from build123d import *

# Parameters (mm, degrees)
SKETCH_1_W          = 38
SKETCH_1_H          = 20
EXTRUDE_1_DEPTH     = 10
SKETCH_2_R          = 2.025
CUT_EXTRUDE_1_DEPTH = 30.342801502
FILLET_1_R          = 0.5
SKETCH_3_R          = 2.5
CUT_EXTRUDE_2_DEPTH = 30.342801604
FILLET_2_R          = 1.5


with BuildPart() as part:
    # 草图1 → 凸台-拉伸1 (new, symmetric)
    with BuildSketch(Plane.XY):
        Rectangle(SKETCH_1_W, SKETCH_1_H)
        with BuildLine():
            Line((2.601020514, 1), (-2.601020514, 1))
            ThreePointArc((-2.601020514, 1), (-12.5, 0), (-2.601020514, -1))
            Line((-2.601020514, -1), (2.601020514, -1))
            ThreePointArc((2.601020514, -1), (12.5, 0), (2.601020514, 1))
        make_face(mode=Mode.SUBTRACT)
    extrude(amount=EXTRUDE_1_DEPTH, both=True)

    # 草图2 → 切除-拉伸1 (cut, through all)
    with BuildSketch(Plane(origin=(0, 10, 0), x_dir=(1, 0, 0), z_dir=(0, 1, 0))):
        with Locations(Location((-7.5, 0, 0), (0, 0, 180))):
            Circle(SKETCH_2_R)
        with Locations(Location((7.5, 0, 0), (0, 0, 180))):
            Circle(SKETCH_2_R)
    extrude(amount=-CUT_EXTRUDE_1_DEPTH, mode=Mode.SUBTRACT)

    # 圆角1
    fillet_1_edges = [part.edges().sort_by_distance(p)[0] for p in [
        (2.601020514, -1, 0),
        (2.601020514, 1, 0),
        (-2.601020514, 1, 0),
        (-2.601020514, -1, 0),
    ]]
    fillet(fillet_1_edges, radius=FILLET_1_R)

    # 草图3 → 切除-拉伸2 (cut, through all)
    with BuildSketch(Plane.XY.offset(10)):
        with Locations((0, 10)):
            Circle(SKETCH_3_R)
        with Locations((0, -10)):
            Circle(SKETCH_3_R)
    extrude(amount=-CUT_EXTRUDE_2_DEPTH, mode=Mode.SUBTRACT)

    # 圆角2
    fillet_2_edges = [part.edges().sort_by_distance(p)[0] for p in [
        (19, 0, 10),
        (-19, 0, 10),
        (19, 0, -10),
        (-19, 0, -10),
    ]]
    fillet(fillet_2_edges, radius=FILLET_2_R)


solid = part.part
Could you check a few things on this model? Use its own coordinates, in mm. A direction names the side the tool comes from. Give positions to 0.01 mm unless a question says otherwise; leave off trailing zeros. Order: outer loops, then holes, each group sorted by start corner. A loop starts at its lowest first (then second) coordinate and runs counter-clockwise, first axis right, second up. Notation, with made-up numbers: (64.5, 59.5) - (90.5, 59.5) arc R32 cw to (90.5, 85.5) - close; hole circle Ø8 at (-17, 84.25). An arc over 180 degrees is marked (long way). Return JSON: item names as keys, results as strings. Group by question number.
Q1. Which directions (+Z, -Z, +X, -X, +Y, -Y) give clear straight access to the entire face, cutting with the end or side of a thin tool? Please do faces 4 (the face through (7.76, 7.32, 2.01)), 5 (the face through (0, 1, 0)).
Q2. Thinking about a two-plate mould opening in Y: for faces 1 (the face through (0, -1, 0)), 2 (the face through (11, 10, 0)), 3 (the face through (-18.57, 0.14, 9.55)), which applies, pulls with the +Y half, pulls with the -Y half, needs draft (parallel to the pull), parting line crosses it, or undercut?
Q3. Will these pins go through, and if not, where does the flat tip stop? pin 1 Ø3.5 at (x, z) = (-0.5, 1.5) entering from +Y; pin 2 Ø2 at (x, z) = (0, -2) entering from -Y.
Q4. Suppose I cut it at C-C, the plane y = 8.5. Please give me the cut outline in (x, z) (3 decimals), and give its area (3 significant figures).
Q5. Suppose I cut it at B-B, the plane y = 0. Please give me the cut outline in (x, z).
Q6. Suppose I cut it at A-A, the plane x = 0. Please give me the cut outline in (y, z), and give its area (3 significant figures).
Q7. Suppose I cut it at D-D, the plane z = 2.75. Please give me the cut outline in (x, y).
Q8. Please list where these lines run through material, in increasing order: line 1 along X through (y, z) = (7.1, 0) (3 decimals); line 2 along X through (y, z) = (-8.5, 0) (3 decimals); line 3 along X through (y, z) = (3.5, -6.25). Write a range as [from, to].
Resolved:
{
 "1": {"face 4": "+Y, -Y", "face 5": "+Z, -Z"},
 "2": {"face 1": "undercut", "face 2": "pulls with the +Y half", "face 3": "needs draft"},
 "3": {"pin 1": "stops at y = 8.91", "pin 2": "stops at y = -7.71"},
 "4": {"outline": "(-19, -8.5) arc R1.5 ccw to (-17.5, -10) - (-2, -10) - (-2, 10) - (-17.5, 10) arc R1.5 ccw to (-19, 8.5) - close; (2, -10) - (17.5, -10) arc R1.5 ccw to (19, -8.5) - (19, 8.5) arc R1.5 ccw to (17.5, 10) - (2, 10) - close; hole circle Ø4.05 at (-7.5, 0); hole circle Ø4.05 at (7.5, 0)", "area": "652 mm2"},
 "5": {"outline": "(-19, -8.5) arc R1.5 ccw to (-17.5, -10) - (-12.5, -10) - (-12.5, 10) - (-17.5, 10) arc R1.5 ccw to (-19, 8.5) - close; (12.5, -10) - (17.5, -10) arc R1.5 ccw to (19, -8.5) - (19, 8.5) arc R1.5 ccw to (17.5, 10) - (12.5, 10) - close"},
 "6": {"outline": "(-7.5, -10) - (-1, -10) - (-1, 10) - (-7.5, 10) - close; (1, -10) - (7.5, -10) - (7.5, 10) - (1, 10) - close", "area": "260 mm2"},
 "7": {"outline": "(-19, -10) - (-2.5, -10) arc R2.5 cw to (2.5, -10) - (19, -10) - (19, 10) - (2.5, 10) arc R2.5 cw to (-2.5, 10) - (-19, 10) - close; hole (-2.69, -1.36) arc R0.5 cw to (-2.21, -1) - (2.21, -1) arc R0.5 cw to (2.69, -1.36) arc R5 ccw (long way) to (2.69, 1.36) arc R0.5 cw to (2.21, 1) - (-2.21, 1) arc R0.5 cw to (-2.69, 1.36) arc R5 ccw (long way) to start"},
 "8": {"line 1": "x = [-19, -9.525], [-5.475, 5.475], [9.525, 19]", "line 2": "x = [-19, -9.525], [-5.475, -2], [2, 5.475], [9.525, 19]", "line 3": "x = [-19, -11.07], [-3.93, 3.93], [11.07, 19]"}
}
